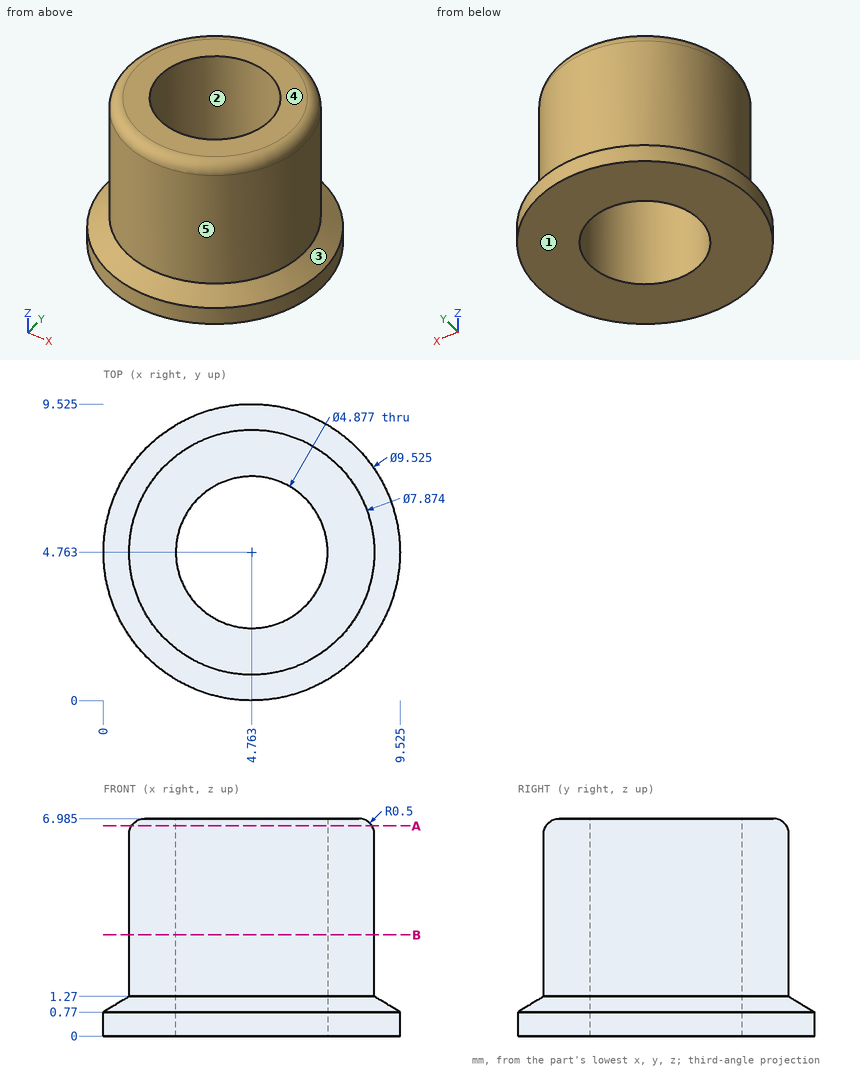
Answer from the drawing. Dimensions are ordinates in mm from the lowest x, y and z of the part. A direction names the side the tool comes from. Give positions to 0.01 mm unless a question says otherwise; leave off trailing zeros. Order: outer loops, then holes, each group sorted by start corner. A loop starts at its lowest first (then second) coordinate and runs counter-clockwise, first axis right, second up.
Item 1: Find the intervals of material crossed by probe 1 along X at (y, z) = (4.75, 5) (1 decimal); probe 2 along X at (y, z) = (4.25, 6) (1 decimal); probe 3 along Y at (x, z) = (7, 6.75) (1 decimal), in increasing order.
From the geometry:
probe 1: x = 0.8 to 2.3, 7.2 to 8.7
probe 2: x = 0.9 to 2.4, 7.1 to 8.7
probe 3: y = 1.6 to 3.8, 5.7 to 7.9
Item 2: Given pin 1 Ø4 at (y, z) = (8, 4.5) entering from +X; pin 2 Ø4 at (x, y) = (5, 7.5) entering from -Z, each flat-ended and moving along its own axis, determine where each tip first touches the part or whether it passes through.
From the geometry:
pin 1: stops at x = 8.5
pin 2: stops at z = 0
Item 3: For a pull along Y with two mould halves and no side action, classify the marked faces 1, 2 and 3 as pulls with the +Y half, pulls with the -Y half, needs draft (parallel to the pull), parting line crosses it, or undercut.
From the geometry:
face 1: needs draft
face 2: undercut
face 3: parting line crosses it
Item 4: The part is cut by section A-A, the plane z = 6.75. Give the vertices of the cut face in (x, y).
From the geometry:
outline: circle Ø7.72 at (4.76, 4.76); hole circle Ø4.88 at (4.76, 4.76)
Item 5: Which of the six approach directions +Z, -Z, +X, -X, +Y, -Y give full straight-line access (tool end or side, diameter ignored) to the marked faces 4 and 5?
From the geometry:
face 4: +Z, +X, -X, +Y, -Y
face 5: +Z
Item 6: The part is cut by section B-B, the plane z = 3.25. Give the vertices of the cut face in (x, y) (1 decimal).
From the geometry:
outline: circle Ø7.9 at (4.8, 4.8); hole circle Ø4.9 at (4.8, 4.8)
